Verification items for the finished model (mm, model axes). A direction names the side the tool comes from. Round coordinates to 2 decimals unless told otherwise and drop trailing zeros. Order: outer loops, then holes, each group sorted by start corner. A loop starts at its lowest first (then second) coordinate and runs counter-clockwise, first axis right, second up. Notation, with made-up numbers: (40.5, 78.25) -> (47.5, 78.25) arc R4 ccw to (47.5, 85.25) -> close; hole circle Ø8 at (-39, -34.5). An arc over 180 degrees is marked (long way). Return JSON: item names as keys, results as strings. Group by question number.
Item 1: Access from +Z, -Z, +X, -X, +Y, -Y to the whole of each face (thin tool, end or side, straight path). Record for faces 1 (the cylindrical face through (3.1, -200.05, 2.96)), 2 (the cylindrical face through (-3.35, -240.758, 2.958)), 3 (the flat face through (-10.3, -225, 3)).
Item 2: Sectioned sample at C-C on x = -23.3. Record the cut outline in (y, z).
Item 3: Sectioned sample at A-A on x = -3.3. Record the cut outline in (y, z), plus the area to 3 significant figures.
Item 4: Sectioned sample at B-B on y = -250. Record the cut outline in (x, z), plus the area to 3 significant figures.
Item 5: Sectioned sample at D-D on z = 5.15. Record the cut outline in (x, y), plus the area to 3 significant figures.
Item 6: Scan lines: probe 1 along Y at (x, z) = (-3.3, 2.8); probe 2 along X at (y, z) = (-254.5, 4.8); probe 3 along Y at (x, z) = (-23.3, 4.75). Record each from-to range of solid material in increasing order. Write a range as from..to.
Item 7: Depth check by flat-ended pin: pin 1 Ø3 at (y, z) = (-242, 1.5) entering from -X. Enter the tip coordinate at first touch or a pass-through.
Item 8: Draft check along Y on faces 4 (the flat face through (3.7, -235, 3)), 5 (the cylindrical face through (-3.25, -265.48, 2.96)), 6 (the cylindrical face through (-27.73, -249.61, 2.96)), 7 (the cylindrical face through (-27.699, -266.437, 2.958)). Enter one of: pulls with the +Y half, pulls with the -Y half, needs draft (parallel to the pull), parting line crosses it, or undercut.
Autodesk Inventor part; units mm, degrees
ref_plane "YZ Plane" through (0, 0, 0) normal (1, 0, 0) x (0, 1, 0)
ref_plane "XZ Plane" through (0, 0, 0) normal (0, 1, 0) x (-1, 0, 0)
ref_plane "XY Plane" through (0, 0, 0) normal (0, 0, 1) x (1, 0, 0)
ref_plane "РабПлоскость1" through (0, 0, 0) normal (0, 0, 1) x (1, 0, 0)
sketch "Эскиз1" plane through (0, 0, 0) normal (0, 0, 1) x (1, 0, 0)
  line L0 (-10.3, -267.007) -> (3.7, -267.007)
  line L1 (-26.3, -267.007) -> (-10.3, -267.007)
  arc A0 (-28.3, -265.007) -> (-26.3, -267.007) centre (-26.3, -265.007) ccw
  line L2 (-28.3, -251.007) -> (-28.3, -265.007)
  arc A1 (-26.3, -249.007) -> (-28.3, -251.007) centre (-26.3, -251.007) ccw
  line L3 (-10.3, -249.007) -> (-26.3, -249.007)
  line L4 (-10.3, -201.4771) -> (-10.3, -249.007)
  arc A2 (-8.3, -199.4771) -> (-10.3, -201.4771) centre (-8.3, -201.4771) ccw
  line L5 (1.7, -199.4771) -> (-8.3, -199.4771)
  arc A3 (3.7, -201.4771) -> (1.7, -199.4771) centre (1.7, -201.4771) ccw
  line L6 (3.7, -267.007) -> (3.7, -201.4771)
  line L7 (3.7, -267.007) -> (-10.3, -267.007)
  line L8 (-1.0506, -258.007) -> (-1.0506, -243.007)
  line L9 (-5.5498, -258.007) -> (-5.5498, -243.007)
  arc A4 (-1.0506, -243.007) -> (-5.5498, -243.007) centre (-3.3002, -243.007) ccw
  arc A5 (-5.5498, -263.1742) -> (-1.0506, -263.1742) centre (-3.3002, -263.2319) ccw
  line L10 (-5.5498, -263.2896) -> (-5.5498, -258.007)
  line L11 (-1.0506, -263.2896) -> (-1.0506, -258.007)
  circle A6 centre (-23.3, -258.4837) radius 2.25
  circle A7 centre (-3.3, -238.0001) radius 1.25
  circle A8 centre (-3.3, -223.0001) radius 1.25
  point P0 (0, 0)
  dimension "d2" = 15
extrude "Выдавливание1" add sketch "Эскиз1" along normal blind 6
sketch "Эскиз2" plane through (0, 0, 0) normal (0, 0, -1) x (-1, 0, 0)
  line L0 (10.3, -225.242) -> (-3.7, -225.242)
  circle A0 centre (3.3, -238.0001) radius 1.25
  circle A1 centre (3.3, -229.8361) radius 1.25
  line L1 (26.3, -267.007) -> (-3.7, -267.007)
  arc A2 (26.3, -267.007) -> (28.3, -265.007) centre (26.3, -265.007) ccw
  line L2 (28.3, -251.007) -> (28.3, -265.007)
  arc A3 (28.3, -251.007) -> (26.3, -249.007) centre (26.3, -251.007) ccw
  line L3 (10.3, -249.007) -> (26.3, -249.007)
  circle A4 centre (23.3, -258.4837) radius 2.25
  line L4 (1.0506, -243.007) -> (1.0506, -263.1742)
  arc A5 (5.5498, -243.007) -> (1.0506, -243.007) centre (3.3002, -243.007) ccw
  line L5 (5.5498, -263.1742) -> (5.5498, -243.007)
  arc A6 (1.0506, -263.1742) -> (5.5498, -263.1742) centre (3.3002, -263.2319) ccw
  line L6 (-3.7, -225.242) -> (-3.7, -267.007)
  line L7 (10.3, -249.007) -> (10.3, -225.242)
  point P0 (0, 0)
properties part number "крепление ремня"
Recorded:
{
 "1": {"face 1": "+Z, -Z, +X, +Y", "face 2": "+Z, -Z", "face 3": "+Z, -Z, -X, +Y"},
 "2": {"outline": "(-267.01, 0) -> (-260.73, 0) -> (-260.73, 6) -> (-267.01, 6) -> close; (-256.23, 0) -> (-249.01, 0) -> (-249.01, 6) -> (-256.23, 6) -> close"},
 "3": {"outline": "(-267.01, 0) -> (-265.48, 0) -> (-265.48, 6) -> (-267.01, 6) -> close; (-240.76, 0) -> (-239.25, 0) -> (-239.25, 6) -> (-240.76, 6) -> close; (-236.75, 0) -> (-224.25, 0) -> (-224.25, 6) -> (-236.75, 6) -> close; (-221.75, 0) -> (-199.48, 0) -> (-199.48, 6) -> (-221.75, 6) -> close", "area": "227 mm²"},
 "4": {"outline": "(-28.03, 0) -> (-5.55, 0) -> (-5.55, 6) -> (-28.03, 6) -> close; (-1.05, 0) -> (3.7, 0) -> (3.7, 6) -> (-1.05, 6) -> close", "area": "163 mm²"},
 "5": {"outline": "(-28.3, -265.01) arc R2 ccw to (-26.3, -267.01) -> (3.7, -267.01) -> (3.7, -201.48) arc R2 ccw to (1.7, -199.48) -> (-8.3, -199.48) arc R2 ccw to (-10.3, -201.48) -> (-10.3, -249.01) -> (-26.3, -249.01) arc R2 ccw to (-28.3, -251.01) -> close; hole circle Ø4.5 at (-23.3, -258.48); hole (-5.55, -263.17) arc R2.25 ccw (long way) to (-1.05, -263.17) -> (-1.05, -243.01) arc R2.25 ccw to (-5.55, -243.01) -> close; hole circle Ø2.5 at (-3.3, -238); hole circle Ø2.5 at (-3.3, -223)", "area": "1,130 mm²"},
 "6": {"probe 1": "-267.01..-265.48, -240.76..-239.25, -236.75..-224.25, -221.75..-199.48", "probe 2": "-28.3..-5.55, -1.05..3.7", "probe 3": "-267.01..-260.73, -256.23..-249.01"},
 "7": {"pin 1": "x = -10.3"},
 "8": {"face 4": "needs draft", "face 5": "undercut", "face 6": "pulls with the +Y half", "face 7": "pulls with the -Y half"}
}
